Part model, mm, in its own coordinate system. Coordinates: 2 decimals unless noted, no trailing zeros. Use a Markdown table: item, result. Add a question column.
1) Wall check: L1, parallel to X at y = 5.75, z = 0; L2, parallel to X at y = 7.8, z = 0; L3, parallel to X at y = 5.5, z = 21.5. Give the ranges that are in metal, low to high. Write a range as [from, to].
2) Two-plate mould, pull along X, no slides. Class faces 1 (the face through (10.99, 8.01, -249.76)), 2 (the face through (146.763, 4.93, -230.195)), 3 (the face through (120, 10, 221)): +X half, -X half, draft (parallel to the pull), parting line (faces both ways), or undercut.
3) Drop flat-ended pins along their axis: P1, Ø2, axis at x = 205.5, y = 3, coming from the +Z side; P2, Ø1.5, axis at x = 39.5, y = 4.5, coming from the +Z side; P3, Ø10, axis at x = 0, z = -261, coming from the -Y side; P4, Ø6, axis at x = -49, y = 2.5, coming from the -Z side. Give the stop position or say it passes through.
4) Saw through at A-A on y = 4.5. Count the separate pieces of the cut face and the enclosed holes in it, then the cut area to 3 significant figures.
```python
from build123d import *

# Parameters (mm, degrees)
BOSS_EXTRUDE1_OUTLINE_R   = 273
BOSS_EXTRUDE1_OUTLINE_R_2 = 4.25
BOSS_EXTRUDE1_OUTLINE_R_3 = 248
BOSS_EXTRUDE1_DEPTH       = 10
SKETCH2_R                 = 250
CUT_EXTRUDE1_DEPTH        = 3
CHAMFER1_SIZE             = 1


# Read off the part's stored shape, not the designer's step: Boss-Extrude1
with BuildPart() as part:
    # Boss-Extrude1 outline → Boss-Extrude1 (new body)
    with BuildSketch(Plane(origin=(0, 0, 0), x_dir=(1, 0, 0), z_dir=(0, 1, 0))):
        Circle(BOSS_EXTRUDE1_OUTLINE_R)
        with Locations((-184.55486989, -184.55486989)):
            Circle(BOSS_EXTRUDE1_OUTLINE_R_2, mode=Mode.SUBTRACT)
        with Locations((0, -261)):
            Circle(BOSS_EXTRUDE1_OUTLINE_R_2, mode=Mode.SUBTRACT)
        with Locations((184.55486989, -184.55486989)):
            Circle(BOSS_EXTRUDE1_OUTLINE_R_2, mode=Mode.SUBTRACT)
        with Locations((-261, 0)):
            Circle(BOSS_EXTRUDE1_OUTLINE_R_2, mode=Mode.SUBTRACT)
        with Locations((-184.55486989, 184.55486989)):
            Circle(BOSS_EXTRUDE1_OUTLINE_R_2, mode=Mode.SUBTRACT)
        Circle(BOSS_EXTRUDE1_OUTLINE_R_3, mode=Mode.SUBTRACT)
        with Locations((261, 0)):
            Circle(BOSS_EXTRUDE1_OUTLINE_R_2, mode=Mode.SUBTRACT)
        with Locations((0, 261)):
            Circle(BOSS_EXTRUDE1_OUTLINE_R_2, mode=Mode.SUBTRACT)
        with Locations((184.55486989, 184.55486989)):
            Circle(BOSS_EXTRUDE1_OUTLINE_R_2, mode=Mode.SUBTRACT)
    extrude(amount=BOSS_EXTRUDE1_DEPTH)

    # Sketch2 → Cut-Extrude1 (cut)
    with BuildSketch(Plane(origin=(0, 10, 0), x_dir=(1, 0, 0), z_dir=(0, 1, 0))):
        with Locations(Location((0, 0, 0), (0, 0, 270))):
            Circle(SKETCH2_R)
    extrude(amount=-CUT_EXTRUDE1_DEPTH, mode=Mode.SUBTRACT)

    # Chamfer1
    chamfer1_edges = [part.edges().sort_by_distance(p)[0] for p in [
        (0, 10, -250),
    ]]
    chamfer(chamfer1_edges, length=CHAMFER1_SIZE)


solid = part.part
```
Results are:
| question | item | result |
|---|---|---|
| 1 | L1 | [-273, -265.25], [-256.75, -248], [248, 256.75], [265.25, 273] |
| 1 | L2 | [-273, -265.25], [-256.75, -250], [250, 256.75], [265.25, 273] |
| 1 | L3 | [-272.15, -247.07], [247.07, 272.15] |
| 2 | face 1 | undercut |
| 2 | face 2 | parting line |
| 2 | face 3 | draft |
| 3 | P1 | z = 180.86 |
| 3 | P2 | z = 270.24 |
| 3 | P3 | y = 0 |
| 3 | P4 | z = -269.1 |
| 4 | separate pieces | 1 |
| 4 | enclosed holes | 9 |
| 4 | area | 40,500 mm2 |
